Design review of the part built by this model. Coordinates are the model's own, in mm. A direction names the side the tool comes from. Give positions to 0.01 mm unless a question says otherwise; leave off trailing zeros. Order: outer loops, then holes, each group sorted by start corner. A loop starts at its lowest first (then second) coordinate and runs counter-clockwise, first axis right, second up. Notation, with made-up numbers: (-31.5, -10.5) -> (21.5, -10.5) arc R26 ccw to (21.5, 10.5) -> close; hole circle Ø8 at (38.25, -23). An arc over 180 degrees is marked (long way). Use a Markdown table: item, result. Add a question column.
Autodesk Inventor part; units mm, degrees
ref_plane "YZ Plane" through (0, 0, 0) normal (1, 0, 0) x (0, 1, 0)
ref_plane "XZ Plane" through (0, 0, 0) normal (0, 1, 0) x (-1, 0, 0)
ref_plane "XY Plane" through (0, 0, 0) normal (0, 0, 1) x (1, 0, 0)
sketch "Sketch1" plane through (0, 0, 0) normal (0, 1, 0) x (-1, 0, 0)
  line L0 (-20, -10) -> (20, -10)
  line L1 (20, -10) -> (20, 10)
  line L2 (20, 10) -> (-20, 10)
  line L3 (-20, 10) -> (-20, -10)
  line L4 (-20, -10) -> (20, 10) construction
  line L5 (20, -10) -> (-20, 10) construction
  circle A0 centre (10, 0) radius 2.6964
  circle A1 centre (24.5, 5) radius 2
  circle A2 centre (24.5, -5) radius 2
  line L6 (66.7, 0) -> (-46.7, 0)
  circle A3 centre (-24.5, 5) radius 2
  circle A4 centre (-24.5, -5) radius 2
  line L7 (50.5, 16) -> (-30.5, 16)
  line L8 (-30.5, 16) -> (-30.5, -16)
  line L9 (-30.5, -16) -> (50.5, -16)
  line L10 (50.5, -16) -> (50.5, 16)
  line L11 (10, 6.1182) -> (10, -6.1182) construction
  line L12 (-28.5, 14.25) -> (-28.5, 16)
  line L13 (20.5, 10.5) -> (20.5, -10.5)
  line L14 (20.5, -10.5) -> (-20.5, -10.5)
  line L15 (-20.5, -10.5) -> (-20.5, 10.5)
  line L16 (-20.5, 10.5) -> (20.5, 10.5)
  point P0 (0, 0)
  point P1 (-20.5, 0)
  point P2 (20.5, 0)
  point P3 (20, 0)
  point P4 (-20, 0)
  dimension "d0" = 40
  dimension "d1" = 20
  dimension "d2" = 30
  dimension "d3" = 10
  dimension "d4" = 4.5
  dimension "d5" = 10
  dimension "d6" = 4.5
  dimension "d7" = 4
  dimension "d8" = 6
  dimension "d9" = 6
  dimension "d31" = 0.5
extrude "Base" add sketch "Sketch1" along normal blind 5.6 contours L15 L14 L13 L6 L10 L9 L8 | L6 L8 L7 L10 L13 L16 L15 | A1 | A2 | A3 | A4
sketch "Sketch3" plane through (0, 5.6, 0) normal (0, 1, 0) x (1, 0, 0)
  line L0 (-66.7, 0) -> (46.7, 0)
  line L1 (0, -6.8326) -> (0, 7.3627) construction
  circle A0 centre (24.5, -5) radius 2.9
  circle A1 centre (24.5, 5) radius 2.9
  circle A2 centre (-24.5, -5) radius 2.9
  circle A3 centre (-24.5, 5) radius 2.9
  line L2 (20, -10) -> (20, 10)
  point P0 (0, 0)
  dimension "d19" = 10
  dimension "d28" = 5.8
  dimension "d32" = 4.5
hole "Servo mount holes" at (24.5, 5.6, 5) at (24.5, 5.6, -5) at (-24.5, 5.6, 5) at (-24.5, 5.6, -5) direction (0, -1, 0) diameter 4.3 end through all counterbore diameter 5.8 counterbore depth 4
sketch "Sketch2" plane through (-50.5, 0, 16) normal (0, 0, 1) x (1, 0, 0)
  line L0 (81, 5.6) -> (0, 5.6)
  line L1 (0, 5.6) -> (12, 5.6)
  line L2 (12, 5.6) -> (12, 18.6)
  line L3 (12, 18.6) -> (0, 18.6)
  line L4 (0, 18.6) -> (0, 5.6)
  circle A0 centre (6, 16.8) radius 3.55
  circle A1 centre (6, 16.8) radius 3.05
  line L5 (40.5, 13.1003) -> (40.5, -16.3877) construction
  line L6 (81, 5.6) -> (69, 5.6)
  line L7 (69, 5.6) -> (69, 18.6)
  line L8 (69, 18.6) -> (81, 18.6)
  line L9 (81, 18.6) -> (81, 5.6)
  circle A2 centre (75, 16.8) radius 3.55
  circle A3 centre (75, 16.8) radius 3.05
  line L10 (2.45, 16.8) -> (9.55, 16.8)
  line L11 (78.55, 16.8) -> (71.45, 16.8)
  point P0 (50.5, 0)
  point P1 (9.0598, 18.6)
  point P2 (2.9402, 18.6)
  point P3 (8.4622, 18.6)
  point P4 (3.5378, 18.6)
  point P5 (6, 18.6)
  point P6 (40.5, 5.6)
  point P7 (75, 18.6)
  point P8 (78.0598, 18.6)
  point P9 (71.9402, 18.6)
  point P10 (72.5378, 18.6)
  point P11 (77.4622, 18.6)
  point P12 (71.95, 16.8)
  point P13 (78.05, 16.8)
  point P14 (9.05, 16.8)
  point P15 (2.95, 16.8)
  dimension "d12" = 12
  dimension "d13" = 13
  dimension "d14" = 7.1
  dimension "d33" = 0.5
  dimension "d38" = 1.8
extrude "Linear rod mount" add sketch "Sketch2" against normal up to surface (32 mm away) contours L0 L4 L3 A0 L2 | L0 L7 L8 A2 L9
extrude "Servo mount hole extended" cut sketch "Sketch3" along normal blind 10 contours A0 | A1
fillet "Fillet1" radius 2 3 edges at (-38.5, 5.6, 0) (18.5, 5.6, 13.25) (18.5, 5.6, -13.25)
fillet "Fillet2" radius 0.5 8 edges at (-50.5, 18.6, 0) (-38.5, 18.6, 0) (18.5, 18.6, 0) (30.5, 18.6, 0) (-47.5598, 18.6, 0) (-41.4402, 18.6, 0) (21.4402, 18.6, 0) (27.5598, 18.6, 0)
sketch "Sketch4" plane through (0, 0, 0) normal (0, 0, 1) x (1, 0, 0)
  line L0 (-50.5, 0) -> (-44.5, 0)
  line L1 (-44.5, 0) -> (-44.5, 10)
  line L2 (-44.5, 10) -> (-50.5, 10)
  line L3 (-50.5, 10) -> (-50.5, 0)
  point P0 (0, 0)
  dimension "d39" = 10
  dimension "d40" = 6
extrude "Extrusion5" add sketch "Sketch4" along normal mid plane 50
fillet "Fillet3" radius 4 4 edges at (-47.5, 10, 25) (-47.5, 0, 25) (-47.5, 10, -25) (-47.5, 0, -25)
sketch "Sketch5" plane through (-44.5, 0, 16) normal (1, 0, 0) x (0, 0, -1)
  arc A0 (-5, 10) -> (-9, 6) centre (-5, 6) ccw
  arc A1 (41, 6) -> (37, 10) centre (37, 6) ccw
  line L0 (-9, 4) -> (-9, 6)
  line L1 (41, 6) -> (41, 4)
  point P0 (16, 0)
  point P1 (-5, 5)
  point P2 (37, 5)
  point P3 (-5, 0)
  point P4 (-9, 5)
  point P5 (41, 5)
hole "Hole2" at (-44.5, 5, 21) at (-44.5, 5, -21) direction (-1, 0, 0) diameter 4.5 end through all counterbore diameter 6 counterbore depth 4
fillet "Fillet4" radius 2 2 edges at (-44.5, 5, 16) (-44.5, 5, -16)
equation "\"d9\" = d8"
properties part number "Servo mount - fron"
1) Add section D-D (z = 11.5). Give the boundary of the cut face in (x, y).
2) The part is to be moulded in two halves that separate along Y. For faces 5 (the cylindrical face through (-49.514, 4.324, 18.854)), 6 (the cylindrical face through (-47.542, 8.797, 23.859)), 7 (the flat face through (-44.5, 4, 24)), say which applies: +Y half, -Y half, draft (parallel to the pull), parting line (faces both ways), or undercut.
3) Insertion check: pin 1 (5.5 mm diameter, centred on x = -45.5, z = 19, fed in from +Y); pin 2 (3 mm diameter, centred on x = -24, z = -6.5, fed in from +Y); pin 3 (9.5 mm diameter, centred on y = 5, z = 21, fed in from +X). Each pin has a flat end and moves straight along its axis. Give the tip position at first contact, or say it passes through.
4) Add section A-A (y = 16.8). Give the boundary of the cut face in (x, z), then the cut area to 3 significant figures.
5) Add section B-B (x = -24.5). Give the boundary of the cut face in (y, z), then the cut area to 3 significant figures.
6) Machinability: for faces 1 (the flat face through (-20.5, 3, 0)), 2 (the flat face through (22, 1.6, 5)), 3 (the flat face through (-44.5, 6, -24)), 4 (the flat face through (-38.5, 13, 0)), which of the approach directions +Z, -Z, +X, -X, +Y, -Y give a long, thin tool a straight path to every point of the face, cutting with its end or side? Answer none if there is none.
7) Add section C-C (x = -10.5). Give the boundary of the cut face in (y, z), then the cut area to 3 significant figures.
8) For L1, parallel to Z at x = 24.5, y = 0.3; L2, parallel to Z at x = -24.5, y = 3.45; L3, parallel to X at y = 16.8, z = 1, list the stretches that pass through material, from the lowest coordinate up. Write a range as [from, to].
Worked answers:
| question | item | result |
|---|---|---|
| 1 | outline | (-50.5, 0) -> (30.5, 0) -> (30.5, 18.1) arc R0.5 ccw to (30, 18.6) -> (28.34, 18.6) arc R0.5 ccw to (27.86, 17.94) arc R3.55 cw (long way) to (21.14, 17.94) arc R0.5 ccw to (20.66, 18.6) -> (19, 18.6) arc R0.5 ccw to (18.5, 18.1) -> (18.5, 7.6) arc R2 cw to (16.5, 5.6) -> (-36.5, 5.6) arc R2 cw to (-38.5, 7.6) -> (-38.5, 18.1) arc R0.5 ccw to (-39, 18.6) -> (-40.66, 18.6) arc R0.5 ccw to (-41.14, 17.94) arc R3.55 cw (long way) to (-47.86, 17.94) arc R0.5 ccw to (-48.34, 18.6) -> (-50, 18.6) arc R0.5 ccw to (-50.5, 18.1) -> close |
| 2 | face 5 | undercut |
| 2 | face 6 | +Y half |
| 2 | face 7 | draft |
| 3 | pin 1 | y = 10 |
| 3 | pin 2 | y = 5.6 |
| 3 | pin 3 | x = -43.47 |
| 4 | outline | (-50.5, -16) -> (-48.05, -16) -> (-48.05, 16) -> (-50.5, 16) -> close; (-40.95, -16) -> (-38.5, -16) -> (-38.5, 16) -> (-40.95, 16) -> close; (18.5, -16) -> (20.95, -16) -> (20.95, 16) -> (18.5, 16) -> close; (28.05, -16) -> (30.5, -16) -> (30.5, 16) -> (28.05, 16) -> close |
| 4 | area | 314 mm^2 |
| 5 | outline | (0, -16) -> (5.6, -16) -> (5.6, -7.9) -> (1.6, -7.9) -> (1.6, -7.15) -> (0, -7.15) -> close; (0, -2.85) -> (1.6, -2.85) -> (1.6, -2.1) -> (5.6, -2.1) -> (5.6, 2.1) -> (1.6, 2.1) -> (1.6, 2.85) -> (0, 2.85) -> close; (0, 7.15) -> (1.6, 7.15) -> (1.6, 7.9) -> (5.6, 7.9) -> (5.6, 16) -> (0, 16) -> close |
| 5 | area | 119 mm^2 |
| 6 | face 1 | +Y, -Y |
| 6 | face 2 | +Y |
| 6 | face 3 | -Z, +X, +Y, -Y |
| 6 | face 4 | +Z, -Z, +Y |
| 7 | outline | (0, -16) -> (5.6, -16) -> (5.6, -10.5) -> (0, -10.5) -> close; (0, 10.5) -> (5.6, 10.5) -> (5.6, 16) -> (0, 16) -> close |
| 7 | area | 61.6 mm^2 |
| 8 | L1 | [-16, -7.15], [-2.85, 2.85], [7.15, 16] |
| 8 | L2 | [-16, -7.9], [-2.1, 2.1], [7.9, 16] |
| 8 | L3 | [-50.5, -48.05], [-40.95, -38.5], [18.5, 20.95], [28.05, 30.5] |
